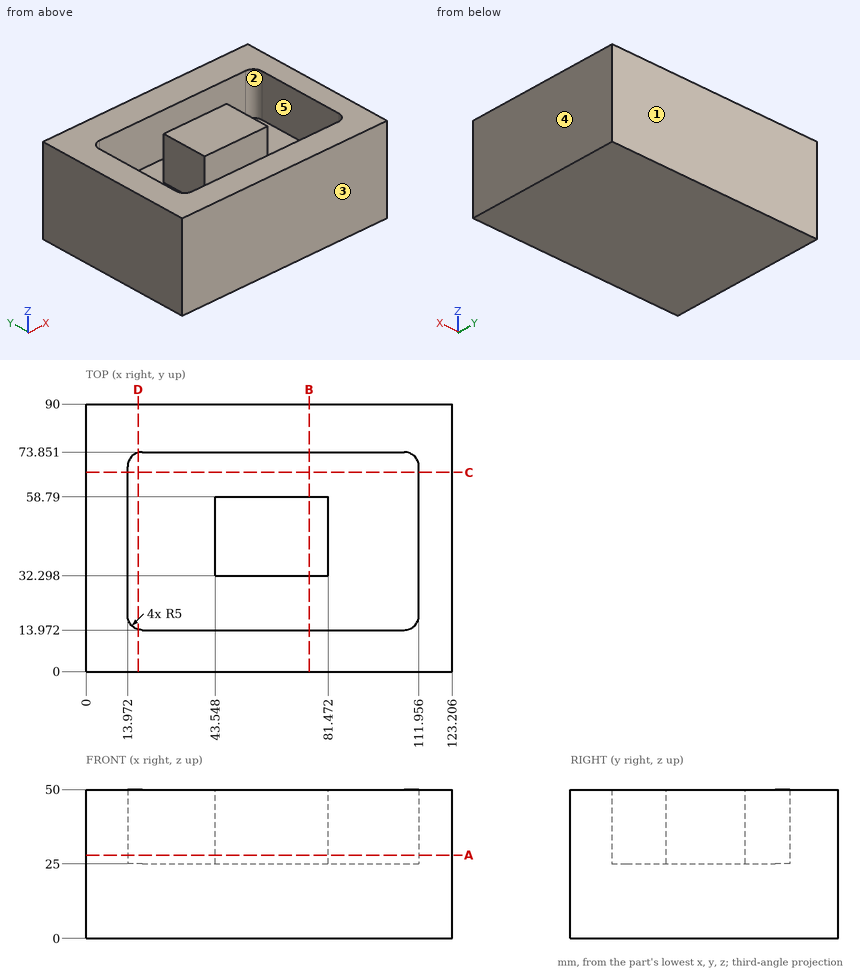
Could you check a few things on this drawing? It's one solid part, dimensions in mm from its lowest x, y, z. A direction names the side the tool comes from. Coordinates: 2 decimals unless noted, no trailing zeros. Order: outer loops, then holes, each group sorted by start corner. A loop starts at its lowest first (then second) coordinate and runs counter-clockwise, first axis right, second up.
1) Which directions (+Z, -Z, +X, -X, +Y, -Y) give clear straight access to the entire face, cutting with the end or side of a thin tool? Please do the marked faces 1 and 2.
2) We'd pull the mould along Y, two halves only. Please class the marked faces 3, 4 and 5: +Y half, -Y half, draft (parallel to the pull), parting line (faces both ways), or undercut.
3) Imagine slicing it at C-C on y = 67. List the corners of the cut face in (x, z) for me (1 decimal).
4) Imagine slicing it at B-B on x = 75. List the corners of the cut face in (y, z) for me, and give its area (3 significant figures).
5) Imagine slicing it at A-A on z = 28. List the corners of the cut face in (x, y) for me (1 decimal).
6) Imagine slicing it at D-D on x = 17.5. List the corners of the cut face in (y, z) for me, and give its area (3 significant figures).
7) I need wall thicknesses on line 1 (X direction, y = 58, z = 39) (1 decimal); line 2 (Y direction, x = 80, z = 47.5); line 3 (Y direction, x = 97.5, z = 26.5). Which ranges of each line are inside material? Lowest first, please.
Response values:
1. face 1: +Z, -Z, +X, -X, +Y
1. face 2: +Z
2. face 3: -Y half
2. face 4: draft
2. face 5: undercut
3. outline: (0, 0) - (123.2, 0) - (123.2, 50) - (112, 50) - (112, 25) - (14, 25) - (14, 50) - (0, 50) - close
4. outline: (0, 0) - (90, 0) - (90, 50) - (73.85, 50) - (73.85, 25) - (58.79, 25) - (58.79, 50) - (32.3, 50) - (32.3, 25) - (13.97, 25) - (13.97, 50) - (0, 50) - close
4. area: 3,670 mm2
5. outline: (0, 0) - (123.2, 0) - (123.2, 90) - (0, 90) - close; (43.5, 32.3) - (81.5, 32.3) - (81.5, 58.8) - (43.5, 58.8) - close; hole (14, 19) arc R5 ccw to (19, 14) - (107, 14) arc R5 ccw to (112, 19) - (112, 68.9) arc R5 ccw to (107, 73.9) - (19, 73.9) arc R5 ccw to (14, 68.9) - close
6. outline: (0, 0) - (90, 0) - (90, 50) - (73.63, 50) - (73.63, 25) - (14.19, 25) - (14.19, 50) - (0, 50) - close
6. area: 3,010 mm2
7. line 1: x = 0 to 14, 43.5 to 81.5, 112 to 123.2
7. line 2: y = 0 to 13.97, 32.3 to 58.79, 73.85 to 90
7. line 3: y = 0 to 13.97, 73.85 to 90
